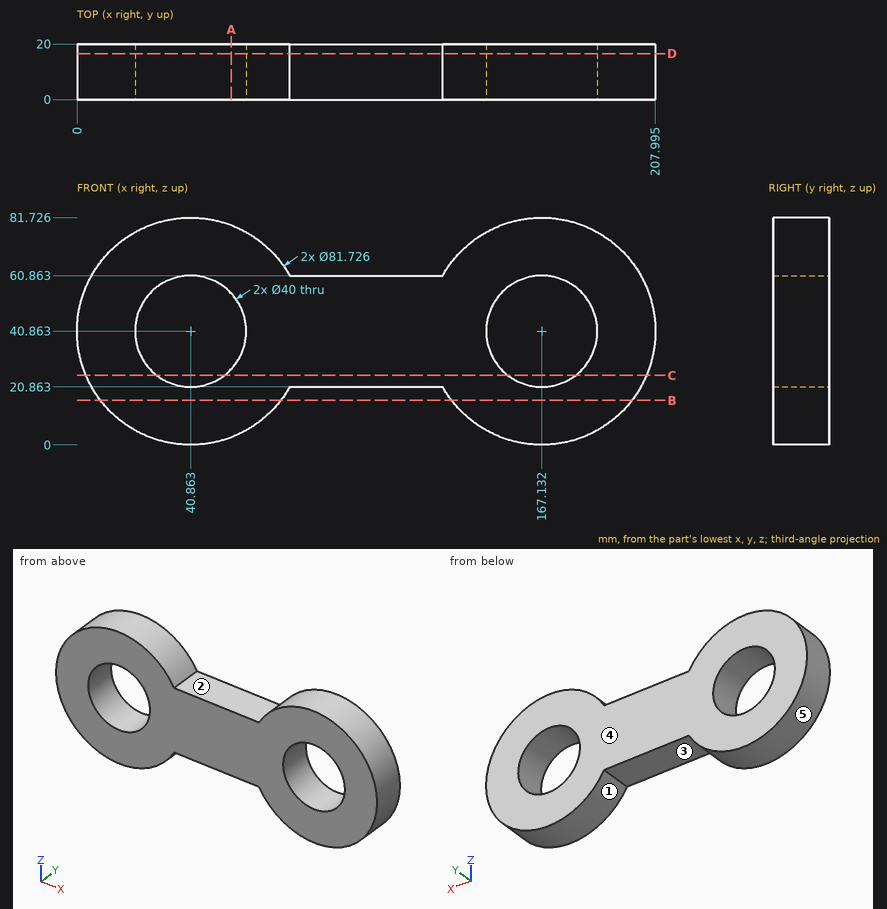
Drawing for the job (mm, zero at the part's lowest x, y, z). A direction names the side the tool comes from. Round coordinates to 2 decimals unless told otherwise and drop trailing zeros. Write each loop counter-clockwise with the first axis right and the second up, starting at its lowest first coordinate (ties: lowest second). Pieces come first, ordered by that corner, then holes. Notation, with made-up numbers: (26, 61.5) - (75, 61.5) arc R18 ccw to (75, 66.5) - close; hole circle Ø7 at (44.25, 21). An arc over 180 degrees is marked (long way). Return JSON: item names as keys, results as strings. Group by question number.
Item 1: Band-saw the part on B-B on z = 16. List the corners of the cut face in (x, y) (1 decimal).
Item 2: Mould opens along X. For the marked faces 4 and 5 say: +X half, -X half, draft (parallel to the pull), parting line (faces both ways), or undercut.
Item 3: 3-axis set-ups, long thin cutter, end or side, ignore diameter. For the marked faces 1, 2 and 3: which of +Z, -Z, +X, -X, +Y, -Y reach the whole face in a straight line?
Item 4: Band-saw the part on C-C on z = 25. List the corners of the cut face in (x, y) (1 decimal).
Item 5: Band-saw the part on A-A on x = 55.5. List the corners of the cut face in (y, z) (1 decimal).
Item 6: Flat gauge pins, fed straight in: pin 1 Ø12 at (x, y) = (158.5, 15) entering from -Z (1 decimal); pin 2 Ø1.5 at (y, z) = (16.5, 56) entering from -X; pin 3 Ø10 at (x, y) = (113, 11) entering from +Z; pin 4 Ø24 at (x, z) = (40.86, 40.86) entering from -Y. Where does each tip first touch, or does it go through?
Item 7: Band-saw the part on D-D on y = 16.5. List the corners of the cut face in (x, z).
Item 8: Probe probe 1 along X at (y, z) = (6, 41) (1 decimal); probe 2 along Z at (x, y) = (168, 17.75) (1 decimal); probe 3 along X at (y, z) = (14.25, 31) (1 decimal). List the from-to ranges inside material, lowest first.
Resolved:
{
 "1": {"outline": "(8.4, 0) - (73.3, 0) - (73.3, 20) - (8.4, 20) - close; (134.7, 0) - (199.6, 0) - (199.6, 20) - (134.7, 20) - close"},
 "2": {"face 4": "draft", "face 5": "undercut"},
 "3": {"face 1": "+Y, -Y", "face 2": "+Z, +Y, -Y", "face 3": "-Z, +Y, -Y"},
 "4": {"outline": "(3.2, 0) - (28.7, 0) - (28.7, 20) - (3.2, 20) - close; (53, 0) - (155, 0) - (155, 20) - (53, 20) - close; (179.3, 0) - (204.8, 0) - (204.8, 20) - (179.3, 20) - close"},
 "5": {"outline": "(0, 2.7) - (20, 2.7) - (20, 27.2) - (0, 27.2) - close; (0, 54.5) - (20, 54.5) - (20, 79) - (0, 79) - close"},
 "6": {"pin 1": "stops at z = 0.1", "pin 2": "stops at x = 2.62", "pin 3": "stops at z = 60.86", "pin 4": "passes through"},
 "7": {"outline": "(76.5, 20.86) - (131.5, 20.86) arc R40.86 ccw (long way) to (131.5, 60.86) - (76.5, 60.86) arc R40.86 ccw (long way) to start; hole circle Ø40 at (40.86, 40.86); hole circle Ø40 at (167.13, 40.86)"},
 "8": {"probe 1": "x = 0 to 20.9, 60.9 to 147.1, 187.1 to 208", "probe 2": "z = 0 to 20.9, 60.8 to 81.7", "probe 3": "x = 1.2 to 23.5, 58.3 to 149.7, 184.5 to 206.8"}
}
